The model under review builds one solid part; all positions refer to its coordinate system, in mm. Round coordinates to 2 decimals unless told otherwise and drop trailing zeros. Order: outer loops, then holes, each group sorted by start corner. A loop starts at its lowest first (then second) coordinate and runs counter-clockwise, first axis right, second up. Notation, with made-up numbers: M 43.5,6.5 L 73.5,6.5 A30 cw 73.5,30.5 Z; hole C 37,-33 d1. An arc over 180 degrees is marked long. Answer as a JSON object with one key per item and string values. Group by question number.
1) To check wall thickness, follow line 1 (Z direction, x = -16.5, y = 13.25); line 2 (X direction, y = 8.5, z = 37); line 3 (X direction, y = 8.75, z = -6). State the ranges of each line that lie inside material, in increasing order.
2) Consider section C-C, the plane y = 13. Write out the cut boundary in (x, z).
3) Insertion check: pin 1 Ø4 at (y, z) = (4.5, 17) entering from +X; pin 2 Ø3 at (y, z) = (5.5, 20.5) entering from -X; pin 3 Ø1.5 at (y, z) = (2, -1) entering from -X. Each pin has a flat end and moves straight along its axis. Give the tip position at first contact, or say it passes through.
4) Consider section A-A, the plane y = 3. Write out the cut boundary in (x, z).
5) Consider section B-B, the plane x = -16.5. Write out the cut boundary in (y, z), then the cut area to 3 significant figures.
```python
from build123d import *

# Parameters (mm, degrees)
SKETCH_1_W          = 89
SKETCH_1_H          = 62
EXTRUDE_1_DEPTH     = 15
CUT_EXTRUDE_START   = -15.000001
SKETCH_2_W          = 114.345269922
SKETCH_2_H          = 82.741202996
CUT_EXTRUDE_2_DEPTH = 15.000002
FILLET_1_R          = 10


with BuildPart() as part:
    # 草图1 → 凸台-拉伸1 (new body)
    with BuildSketch(Plane(origin=(0, 0, 0), x_dir=(1, 0, 0), z_dir=(0, 1, 0))):
        with Locations((-7.7, -10.288888889)):
            Rectangle(SKETCH_1_W, SKETCH_1_H)
    extrude(amount=EXTRUDE_1_DEPTH)

    # 草图2 → 切除-拉伸2 (cut)
    with BuildSketch(Plane(origin=(0, 15, 0), x_dir=(1, 0, 0), z_dir=(0, 1, 0)).offset(CUT_EXTRUDE_START)):
        with Locations((-11.341983823, -7.488413354)):
            Rectangle(SKETCH_2_W, SKETCH_2_H)
        with BuildLine():
            Line((-28.520508076, 20.711111111), (13.120508076, 20.711111111))
            ThreePointArc((13.120508076, 20.711111111), (23.620508076, 17.897644591), (31.307041555, 10.211111111))
            ThreePointArc((31.307041555, 10.211111111), (36.8, -10.288888889), (31.307041555, -30.788888889))
            ThreePointArc((31.307041555, -30.788888889), (23.620508076, -38.475422368), (13.120508076, -41.288888889))
            Line((13.120508076, -41.288888889), (-28.520508076, -41.288888889))
            ThreePointArc((-28.520508076, -41.288888889), (-39.020508076, -38.475422368), (-46.707041555, -30.788888889))
            ThreePointArc((-46.707041555, -30.788888889), (-52.2, -10.288888889), (-46.707041555, 10.211111111))
            ThreePointArc((-46.707041555, 10.211111111), (-39.020508076, 17.897644591), (-28.520508076, 20.711111111))
        make_face(mode=Mode.SUBTRACT)
    extrude(amount=CUT_EXTRUDE_2_DEPTH, mode=Mode.SUBTRACT)

    # 圆角1
    fillet_1_edges = [part.edges().sort_by_distance(p)[0] for p in [
        (23.620508076, 15, 38.475422368),
        (36.8, 15, 10.288888889),
        (-52.2, 15, 10.288888889),
        (-39.020508076, 15, -17.897644591),
        (-7.7, 15, 41.288888889),
        (-39.020508076, 15, 38.475422368),
        (-7.7, 15, -20.711111111),
        (23.620508076, 15, -17.897644591),
    ]]
    fillet(fillet_1_edges, radius=FILLET_1_R)


solid = part.part
```
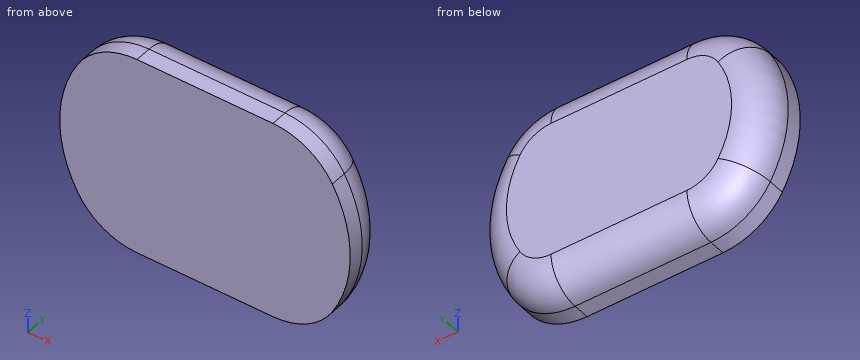
Results list:
{
 "1": {"line 1": "-16.36 to 36.94", "line 2": "-40.16 to 24.76", "line 3": "-48.03 to 32.63"},
 "2": {"outline": "M -43.24,-8.21 A17 ccw -28.52,-16.71 L 13.12,-16.71 A17 ccw 27.84,-8.21 A37 ccw 27.84,28.79 A17 ccw 13.12,37.29 L -28.52,37.29 A17 ccw -43.24,28.79 A37 ccw Z"},
 "3": {"pin 1": "x = 36.53", "pin 2": "x = -51.26", "pin 3": "x = -50.82"},
 "4": {"outline": "M -46.71,-10.21 A21 ccw -28.52,-20.71 L 13.12,-20.71 A21 ccw 31.31,-10.21 A41 ccw 31.31,30.79 A21 ccw 13.12,41.29 L -28.52,41.29 A21 ccw -46.71,30.79 A41 ccw Z"},
 "5": {"outline": "M 0,-20.71 L 5,-20.71 A10 ccw 15,-10.71 L 15,31.29 A10 ccw 5,41.29 L 0,41.29 Z", "area": "887 mm^2"}
}
